```python
from build123d import *

# Parameters (mm, degrees)
SKETCH1_R           = 3.5
SKETCH1_W           = 4.25
SKETCH1_H           = 4.25
BOSS_EXTRUDE1_DEPTH = 140


with BuildPart() as part:
    # Sketch1 → Boss-Extrude1 (new, symmetric)
    with BuildSketch(Plane.XY):
        with BuildLine():
            Line((-13, 8), (-9.555634919, 8))
            Line((-9.555634919, 8), (-5.276706211, 3.721071292))
            ThreePointArc((-5.276706211, 3.721071292), (-4.996490762, 3.172693256), (-5.090706575, 2.564119062))
            ThreePointArc((-5.090706575, 2.564119062), (-5.688941006, -0.354894676), (-4.732561446, -3.176926527))
            Line((-4.732561446, -3.176926527), (-9.555634919, -8))
            Line((-9.555634919, -8), (-13, -8))
            Line((-13, -8), (-13, -4.1))
            Line((-13, -4.1), (-14.3, -4.1))
            Line((-14.3, -4.1), (-14.3, -4.8))
            Line((-14.3, -4.8), (-15, -4.8))
            Line((-15, -4.8), (-15, -15))
            Line((-15, -15), (-4.1, -15))
            Line((-4.1, -15), (-4.1, -13))
            Line((-4.1, -13), (-8, -13))
            Line((-8, -13), (-8, -9.555634919))
            Line((-8, -9.555634919), (-3.721071292, -5.276706211))
            ThreePointArc((-3.721071292, -5.276706211), (-3.172693256, -4.996490762), (-2.564119062, -5.090706575))
            ThreePointArc((-2.564119062, -5.090706575), (0, -5.7), (2.564119062, -5.090706575))
            ThreePointArc((2.564119062, -5.090706575), (3.172693256, -4.996490762), (3.721071292, -5.276706211))
            Line((3.721071292, -5.276706211), (8, -9.555634919))
            Line((8, -9.555634919), (8, -13))
            Line((8, -13), (4.1, -13))
            Line((4.1, -13), (4.1, -15))
            Line((4.1, -15), (15, -15))
            Line((15, -15), (15, -4.8))
            Line((15, -4.8), (14.3, -4.8))
            Line((14.3, -4.8), (14.3, -4.1))
            Line((14.3, -4.1), (13, -4.1))
            Line((13, -4.1), (13, -8))
            Line((13, -8), (9.555634919, -8))
            Line((9.555634919, -8), (5.276706211, -3.721071292))
            ThreePointArc((5.276706211, -3.721071292), (4.996490762, -3.172693256), (5.090706575, -2.564119062))
            ThreePointArc((5.090706575, -2.564119062), (5.7, 0), (5.090706575, 2.564119062))
            ThreePointArc((5.090706575, 2.564119062), (4.996490762, 3.172693256), (5.276706211, 3.721071292))
            Line((5.276706211, 3.721071292), (9.555634919, 8))
            Line((9.555634919, 8), (13, 8))
            Line((13, 8), (13, 4.1))
            Line((13, 4.1), (14.3, 4.1))
            Line((14.3, 4.1), (14.3, 4.8))
            Line((14.3, 4.8), (15, 4.8))
            Line((15, 4.8), (15, 15))
            Line((15, 15), (4.1, 15))
            Line((4.1, 15), (4.1, 13))
            Line((4.1, 13), (8, 13))
            Line((8, 13), (8, 9.555634919))
            Line((8, 9.555634919), (3.721071292, 5.276706211))
            ThreePointArc((3.721071292, 5.276706211), (3.172693256, 4.996490762), (2.564119062, 5.090706575))
            ThreePointArc((2.564119062, 5.090706575), (0, 5.7), (-2.564119062, 5.090706575))
            ThreePointArc((-2.564119062, 5.090706575), (-3.172693256, 4.996490762), (-3.721071292, 5.276706211))
            Line((-3.721071292, 5.276706211), (-8, 9.555634919))
            Line((-8, 9.555634919), (-8, 13))
            Line((-8, 13), (-4.1, 13))
            Line((-4.1, 13), (-4.1, 15))
            Line((-4.1, 15), (-15, 15))
            Line((-15, 15), (-15, 4.8))
            Line((-15, 4.8), (-14.3, 4.8))
            Line((-14.3, 4.8), (-14.3, 4.1))
            Line((-14.3, 4.1), (-13, 4.1))
            Line((-13, 4.1), (-13, 8))
        make_face()
        Circle(SKETCH1_R, mode=Mode.SUBTRACT)
        with Locations((11.375, 11.375)):
            Rectangle(SKETCH1_W, SKETCH1_H, mode=Mode.SUBTRACT)
        with Locations((-11.375, -11.375)):
            Rectangle(SKETCH1_W, SKETCH1_H, mode=Mode.SUBTRACT)
        with Locations((11.375, -11.375)):
            Rectangle(SKETCH1_W, SKETCH1_H, mode=Mode.SUBTRACT)
        with Locations((-11.375, 11.375)):
            Rectangle(SKETCH1_W, SKETCH1_H, mode=Mode.SUBTRACT)
    extrude(amount=BOSS_EXTRUDE1_DEPTH, both=True)


solid = part.part
```
Check sheet for the modelled part. Datum: model origin and axes. Units: mm. A direction names the side the tool comes from. Give positions to 0.01 mm unless a question says otherwise; leave off trailing zeros. Order: outer loops, then holes, each group sorted by start corner. A loop starts at its lowest first (then second) coordinate and runs counter-clockwise, first axis right, second up. Notation, with made-up numbers: (-21, 62) -> (-8, 62) arc R25 cw to (-8, 82) -> close; hole circle Ø1 at (-1, 81). An arc over 180 degrees is marked (long way). Return JSON: item names as keys, results as strings.
1. Set-up check for faces 1 (the cylindrical face through (5.7, 0, 2)), 2 (the flat face through (-7.446, 5.89, 1.96)): record each of +Z, -Z, +X, -X, +Y, -Y from which the full face is reachable in a straight line by a thin tool's end or side.
From the geometry:
{"face 1": "+Z, -Z, +X", "face 2": "+Z, -Z"}
2. Cross-section at A-A, the plane y = 0. Record the cut outline in (x, z).
From the geometry:
{"outline": "(-5.7, -140) -> (-3.5, -140) -> (-3.5, 140) -> (-5.7, 140) -> close; (3.5, -140) -> (5.7, -140) -> (5.7, 140) -> (3.5, 140) -> close"}
3. Cross-section at C-C, the plane z = 114. Count the separate pieces of the cut face and the enclosed holes in it, plus the area to 3 significant figures.
From the geometry:
{"separate pieces": "1", "enclosed holes": "5", "area": "303 mm^2"}
4. Mould release check, pull along Y, two halves, no side actions. Record for faces 3 (the flat face through (11, -9.25, 2)), 4 (the flat face through (-10, -15, 2)), 5 (the flat face through (10, 15, 2)): +Y half, -Y half, draft (parallel to the pull), parting line (faces both ways), or undercut.
From the geometry:
{"face 3": "undercut", "face 4": "-Y half", "face 5": "+Y half"}
5. Material ranges on probe 1 along Y at (x, z) = (-0.5, -91.5); probe 2 along X at (y, z) = (13.25, 51); probe 3 along X at (y, z) = (13.75, -8), recorded low to high. Write a range as [from, to].
From the geometry:
{"probe 1": "[-5.68, -3.46], [3.46, 5.68]", "probe 2": "[-15, -13.5], [-9.25, -4.1], [4.1, 9.25], [13.5, 15]", "probe 3": "[-15, -4.1], [4.1, 15]"}
6. Go/stop test with a flat-tipped pin: P1, Ø4, axis at x = 1, z = -47.5, coming from the -Y side. Record where the tip stops, or that it passes through.
From the geometry:
{"P1": "y = -5.7"}
